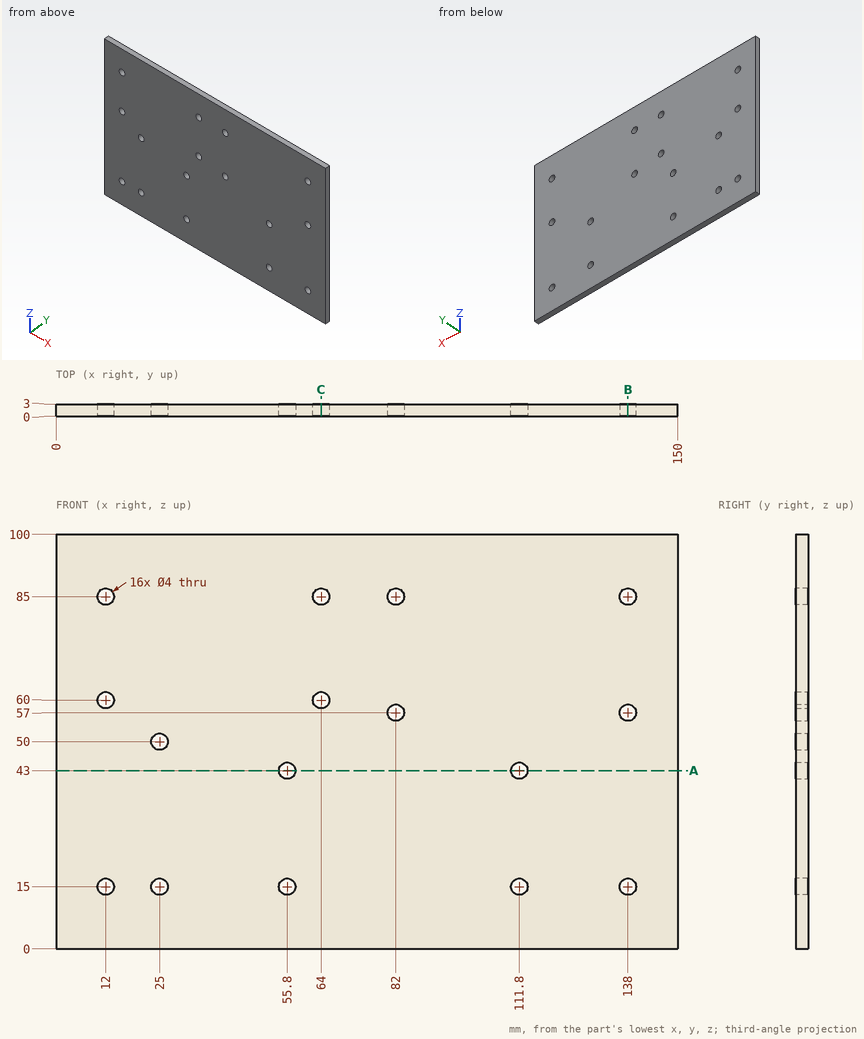
Design review of the part shown in the three views and the two pictorial views. Dimensions are in mm from the part's minimum x, y and z. Coordinates: 2 decimals unless noted, no trailing zeros. Write each loop counter-clockwise with the first axis right and the second up, starting at its lowest first coordinate (ties: lowest second). Pieces come first, ordered by that corner, then holes.
(1) Add section B-B on x = 138. Give the boundary of the cut face in (y, z).
(2) Add section C-C on x = 64. Give the boundary of the cut face in (y, z), then the cut area to 3 significant figures.
(3) For pin 1 Ø3 at (x, z) = (138, 85) entering from -Y, flat-tipped, find the tip position at first contact; note if it passes through.
(4) Wall thickness on probe 1 along X at (y, z) = (1.5, 60); probe 2 along Z at (x, y) = (25, 2.4); probe 3 along X at (y, z) = (2.15, 15): over which ranges is each line inside the solid? List them lowest first.
(5) Add section A-A on z = 43. Give the boundary of the cut face in (x, y), then the cut area to 3 significant figures.
Answer sheet:
1. outline: (0, 0) - (3, 0) - (3, 13) - (0, 13) - close; (0, 17) - (3, 17) - (3, 55) - (0, 55) - close; (0, 59) - (3, 59) - (3, 83) - (0, 83) - close; (0, 87) - (3, 87) - (3, 100) - (0, 100) - close
2. outline: (0, 0) - (3, 0) - (3, 58) - (0, 58) - close; (0, 62) - (3, 62) - (3, 83) - (0, 83) - close; (0, 87) - (3, 87) - (3, 100) - (0, 100) - close
2. area: 276 mm2
3. pin 1: passes through
4. probe 1: x = 0 to 10, 14 to 62, 66 to 150
4. probe 2: z = 0 to 13, 17 to 48, 52 to 100
4. probe 3: x = 0 to 10, 14 to 23, 27 to 53.8, 57.8 to 109.8, 113.8 to 136, 140 to 150
5. outline: (0, 0) - (53.8, 0) - (53.8, 3) - (0, 3) - close; (57.8, 0) - (109.8, 0) - (109.8, 3) - (57.8, 3) - close; (113.8, 0) - (150, 0) - (150, 3) - (113.8, 3) - close
5. area: 426 mm2
